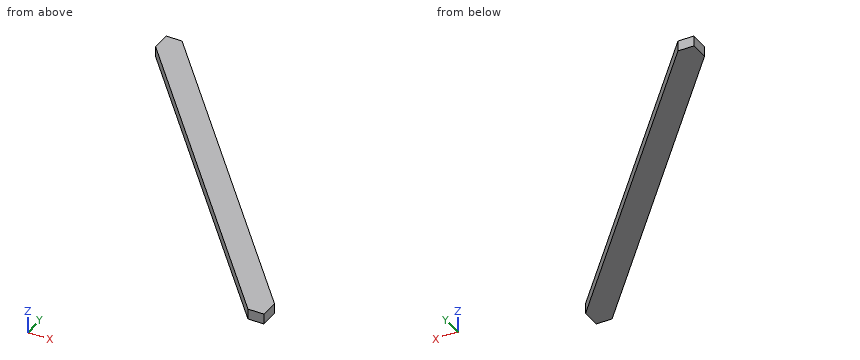
Autodesk Inventor part; units mm, degrees
ref_plane "YZ Plane" through (0, 0, 0) normal (1, 0, 0) x (0, 1, 0)
ref_plane "XZ Plane" through (0, 0, 0) normal (0, 1, 0) x (-1, 0, 0)
ref_plane "XY Plane" through (0, 0, 0) normal (0, 0, 1) x (1, 0, 0)
sketch "Sketch1" plane through (0, 0, 0) normal (0, 0, 1) x (1, 0, 0)
  line L0 (-1041.4, 1219.2) -> (-1041.4, 0)
  line L1 (-1041.4, 1219.2) -> (0, 1219.2)
  line L2 (0, 0) -> (0, 1219.2)
  line L3 (0, 0) -> (-1041.4, 0)
  line L4 (0, 0) -> (0, 68.4388)
  line L5 (0, 68.4388) -> (-982.9419, 1219.2)
  line L6 (-982.9419, 1219.2) -> (-1041.4, 1219.2)
  line L7 (-1041.4, 1219.2) -> (-1041.4, 1150.7612)
  line L8 (-1041.4, 1150.7612) -> (-58.4581, 0)
  line L9 (-58.4581, 0) -> (0, 0)
extrude "Extrusion1" add sketch "Sketch1" against normal blind 38.1 contours L1 L5 L2 L3 L8 L0
properties part number "44x2x4"
Verification items for the finished model (mm, model axes). Give positions to 0.01 mm unless a question says otherwise; leave off trailing zeros. Loops run counter-clockwise (first coordinate to the right, second up) from the corner with the lowest first, then second, coordinate; pieces in that order, holes last. Notation, with made-up numbers: M -25,5.25 L -7,5.25 A11 cw -7,18.25 Z; hole C 72.5,39 d11. An arc over 180 degrees is marked long. Return JSON: item names as keys, results as strings.
1) Gauge pin test, flat ends, axial feed: P1, Ø1.5, axis at x = -337.5, z = -16, coming from the -Y side; P2, Ø5, axis at x = -418, z = -15, coming from the +Y side; P3, Ø10, axis at y = 957.5, z = -11.5, coming from the +X side. Record the tip position at first contact, or that the pin passes through.
Findings:
{"P1": "stops at y = 325.81", "P2": "stops at y = 560.73", "P3": "stops at x = -755.14"}
2) Section check A-A, the plane z = -20. Enter the section's corners in (x, y), and give its area (3 significant figures).
Findings:
{"outline": "M -1041.4,1150.76 L -58.46,0 L 0,0 L 0,68.44 L -982.94,1219.2 L -1041.4,1219.2 Z", "area": "139,000 mm2"}
3) Material ranges on L1, parallel to X at y = 859.5, z = -6.5; L2, parallel to Y at x = -703.5, z = -10; L3, parallel to X at y = 919, z = -26.5, recorded low to high. Write a range as [from, to].
Findings:
{"L1": "x = [-792.61, -675.7]", "L2": "y = [755.17, 892.05]", "L3": "x = [-843.44, -726.52]"}
4) Section check C-C, the plane x = -678. Enter the section's corners in (y, z).
Findings:
{"outline": "M 725.32,-38.1 L 862.19,-38.1 L 862.19,0 L 725.32,0 Z"}
5) Section check B-B, the plane y = 755. Enter the section's corners in (x, z).
Findings:
{"outline": "M -703.35,-38.1 L -586.44,-38.1 L -586.44,0 L -703.35,0 Z"}
